Can you work these out from the model? Positions are in its coordinate system, mm. A direction names the side the tool comes from. Round coordinates to 2 decimals unless told otherwise and drop trailing zeros. Order: outer loops, then holes, each group sorted by start corner. A loop starts at its lowest first (then second) coordinate and runs counter-clockwise, first axis right, second up. Notation, with made-up numbers: M 44.5,62.25 L 100.5,62.25 A19 cw 100.5,82.25 Z; hole C 18.25,73 d10. An arc over 180 degrees is marked long. Answer as a JSON object with one key per item and string values. Group by question number.
Autodesk Inventor part; units mm, degrees
ref_plane "Work Plane1" through (-10, 25, 0) normal (0, 1, 0) x (1, 0, 0)
ref_plane "YZ Plane" through (0, 0, 0) normal (1, 0, 0) x (0, 1, 0)
ref_plane "XZ Plane" through (0, 0, 0) normal (0, 1, 0) x (-1, 0, 0)
sketch "Sketch1" plane through (0, 0, 0) normal (0, 0, 1) x (1, 0, 0)
  line L0 (-10, -25) -> (10, -25)
  line L1 (10, -25) -> (10, 25)
  line L2 (10, 25) -> (-10, 25)
  line L3 (-10, 25) -> (-10, -25)
  line L4 (-10, -25) -> (10, 25) construction
  line L5 (10, -25) -> (-10, 25) construction
  point P0 (0, 0)
  dimension "d0" = 20
  dimension "d1" = 50
ref_plane "Work Plane1" through (-10, 25, 0) normal (0, 1, 0) x (1, 0, 0)
sketch "Sketch2" plane through (-10, 25, 0) normal (0, 1, 0) x (1, 0, 0)
  line L0 (20, 0) -> (0, 0)
  line L1 (0, 0) -> (20, 0)
  line L2 (20, 0) -> (20, -40)
  line L3 (20, -40) -> (0, -40)
  line L4 (0, -40) -> (0, 0)
  point P0 (10, 0)
  dimension "d4" = 40
extrude "Extrusion2" add sketch "Sketch2" along normal blind 5
sketch "Sketch3" plane through (-10, 25, 40) normal (0, 0, 1) x (1, 0, 0)
  line L0 (20, -50) -> (20, 0)
  line L1 (20, 0) -> (0, 0)
  line L2 (0, 0) -> (0, -50)
  line L3 (0, -50) -> (20, -50)
  line L4 (0, 0) -> (20, 0)
  line L5 (20, 0) -> (20, 5)
  line L6 (0, 5) -> (20, 5)
  line L7 (0, 0) -> (0, 5)
  point P0 (10, -25)
extrude "Extrusion3" add sketch "Sketch3" along normal blind 5
extrude "Extrusion4" add sketch "Sketch1" against normal blind 5
sketch "Sketch4" plane through (10, 30, 0) normal (0, 0, -1) x (-1, 0, 0)
  line L0 (0, -5) -> (20, -5)
  line L1 (20, -5) -> (20, 0)
  line L2 (0, 0) -> (20, 0)
  line L3 (0, -5) -> (0, 0)
  point P0 (10, -30)
extrude "Extrusion5" add sketch "Sketch4" along normal blind 5
sketch "Sketch5" plane through (-10, 30, 0) normal (0, 1, 0) x (1, 0, 0)
  circle A0 centre (10, -20) radius 2.6
  point P0 (10, 0)
  dimension "d13" = 5.2
extrude "Extrusion6" cut sketch "Sketch5" against normal blind 10
sketch "Sketch6" plane through (-10, 30, 0) normal (0, 1, 0) x (1, 0, 0)
  line L0 (20, 0) -> (20, 5)
  line L1 (20, 5) -> (30, 5)
  line L2 (30, 5) -> (30, -45)
  line L3 (30, -45) -> (20, -45)
  line L4 (20, -45) -> (20, 5)
  line L5 (20, 5) -> (0, 5)
  line L6 (0, 5) -> (-10, 5)
  line L7 (-10, 5) -> (-10, -45)
  line L8 (-10, -45) -> (0, -45)
  line L9 (0, -45) -> (0, 5)
  point P0 (10, 0)
  dimension "d16" = 10
  dimension "d17" = 50
  dimension "d18" = 10
extrude "Extrusion7" add sketch "Sketch6" against normal blind 5
sketch "Sketch7" plane through (-10, 25, 0) normal (0, -1, 0) x (1, 0, 0)
  line L0 (20, -5) -> (30, -5)
  line L1 (30, -5) -> (20, -5)
  line L2 (20, -5) -> (20, 0)
  line L3 (20, 0) -> (30, 0)
  line L4 (30, 0) -> (30, -5)
  line L5 (30, -5) -> (-10, -5)
  line L6 (0, 0) -> (0, -5)
  line L7 (-10, -5) -> (0, -5)
  line L8 (0, -5) -> (0, 0)
  line L9 (0, 0) -> (-10, 0)
  line L10 (-10, 0) -> (-10, -5)
  line L11 (-10, 45) -> (30, 45)
  line L12 (30, -5) -> (30, 45)
  line L13 (20, 45) -> (30, 45)
  line L14 (30, 45) -> (30, 40)
  line L15 (30, 40) -> (20, 40)
  line L16 (20, 40) -> (20, 45)
  line L17 (-10, 45) -> (0, 45)
  line L18 (0, 45) -> (0, 40)
  line L19 (0, 40) -> (-10, 40)
  line L20 (-10, 40) -> (-10, 45)
  point P0 (10, 0)
  dimension "d21" = 5
extrude "Extrusion8" add sketch "Sketch7" along normal blind 50
properties part number "brazo"
Item 1: If we mould it in two halves opening along Z, with no side actions, what happens to faces 3 (the face through (0, 3, 45)), 4 (the face through (0, 25, 24)), 5 (the face through (-4, 30, 20)), 6 (the face through (0, 0, 40))? For each: +Z half, -Z half, draft (parallel to the pull), parting line (faces both ways), or undercut.
Item 2: Suppose I cut it at A-A, the plane y = -21. Write out the boundary of the cut face in (x, z), and give its area (3 significant figures).
Item 3: Suppose I cut it at D-D, the plane x = 12. Write out the boundary of the cut face in (y, z).
Item 4: Suppose I cut it at C-C, the plane z = 20. Write out the boundary of the cut face in (x, y), and give its area (3 significant figures).
Item 5: Suppose I cut it at B-B, the plane x = 0. Write out the boundary of the cut face in (y, z), and give its area (3 significant figures).
Item 6: I'm going to push a flat-ended pin straight in: pin 1 Ø12 at (x, z) = (-7, 15.5) entering from -Y. Where does the tip first touch, or does it pass through?
Item 7: On a 3-axis mill with a long thin cutter (end or side, diameter ignored), from which of +Z, -Z, +X, -X, +Y, -Y can I reach the whole of each face in a straight line? I mean faces 1 (the face through (0, -25, -2)), 2 (the face through (0, 0, 0)). Say none if no direction works.
Item 8: I need wall thicknesses on line 1 (Z direction, x = -4.5, y = 1); line 2 (Z direction, x = 0, y = 26.3); line 3 (X direction, y = 26, z = 20). Which ranges of each line are inside material? Lowest first, please.
Computed:
{
 "1": {"face 3": "+Z half", "face 4": "undercut", "face 5": "draft", "face 6": "undercut"},
 "2": {"outline": "M -20,-5 L 20,-5 L 20,0 L -20,0 Z; M -20,40 L 20,40 L 20,45 L -20,45 Z", "area": "400 mm^2"},
 "3": {"outline": "M -25,-5 L 30,-5 L 30,45 L -25,45 L -25,40 L 25,40 L 25,0 L -25,0 Z"},
 "4": {"outline": "M -20,25 L -2.6,25 L -2.6,30 L -20,30 Z; M 2.6,25 L 20,25 L 20,30 L 2.6,30 Z", "area": "174 mm^2"},
 "5": {"outline": "M -25,-5 L 30,-5 L 30,17.4 L 25,17.4 L 25,0 L -25,0 Z; M -25,40 L 25,40 L 25,22.6 L 30,22.6 L 30,45 L -25,45 Z", "area": "724 mm^2"},
 "6": {"pin 1": "stops at y = 25"},
 "7": {"face 1": "+Z, -Z, +X, -X, -Y", "face 2": "+X, -X, -Y"},
 "8": {"line 1": "z = -5 to 0, 40 to 45", "line 2": "z = -5 to 17.4, 22.6 to 45", "line 3": "x = -20 to -2.6, 2.6 to 20"}
}
